Model file for the job. Use its own axes, mm. Coordinates: 2 decimals unless noted, no trailing zeros. Write each loop counter-clockwise with the first axis right and the second up, starting at its lowest first coordinate (ties: lowest second). Pieces come first, ordered by that corner, then holes. Notation, with made-up numbers: (-30, 69.5) - (-5, 69.5) arc R7 cw to (-5, 81.5) - close; hole circle Ø10 at (82.5, -15). An arc over 180 degrees is marked (long way). Put each result on its own line as item: value. Start each with the question number.
1. Pull direction Z, two halves, no side cores. Call faces 1 (the face through (-244.27, -2.5, -39.93)), 2 (the face through (-250.948, -2.504, -31.747)), 3 (the face through (-250, 0, -51)): released by +Z, released by -Z, zero draft, split by the parting line, or undercut.
2. Drop flat-ended pins along their axis: P1, Ø4, axis at x = -254.15, z = -32.75, coming from the +Y side; P2, Ø3, axis at x = -239.5, y = -1, coming from the -Z side. Give the stop position or say it passes through.
3. Saw through at D-D, the plane z = -48. Write the cut outline in (x, y), plus the area to 3 significant figures.
4. Saw through at B-B, the plane z = -33.5. Write the cut outline in (x, y).
5. Drill centre lines: L1, parallel to Z at x = -255.5, y = -1.9; L2, parallel to X at y = -3.25, z = -69.5; L3, parallel to Z at x = -252, y = -3.25. Where is each one in solid material? Low to high. Write a range as from..to.
6. Saw through at A-A, the plane x = -249. Write the cut outline in (y, z).
7. Saw through at C-C, the plane y = -1.4. Write the cut outline in (x, z), plus the area to 3 significant figures.
```python
from build123d import *

# Parameters (mm, degrees)
F0_R     = 16.045413
F0_R_2   = 3.352999
F1_DEPTH = 5.08


with BuildPart() as f1:
    # F0 (on Front) → F1 (new body)
    with BuildSketch(Plane.XZ):
        with BuildLine():
            Line((-269.792154, -66.505959), (-268.242146, -61.329008))
            ThreePointArc((-268.242146, -61.329008), (-269.196215, -63.86387), (-269.792154, -66.505959))
        make_face()
        with BuildLine():
            Line((-255.64608, -19.258766), (-268.242146, -61.329008))
            Line((-268.242146, -61.329008), (-269.792154, -66.505959))
            ThreePointArc((-269.792154, -66.505959), (-246.977926, -88.814828), (-233.206555, -60.030735))
            Line((-233.206555, -60.030735), (-255.64608, -19.258766))
        make_face()
        with Locations((-250.397801, -69.492221)):
            Circle(F0_R, mode=Mode.SUBTRACT)
        with Locations((-254.146576, -32.754317)):
            Circle(F0_R_2, mode=Mode.SUBTRACT)
    extrude(amount=F1_DEPTH)


solid = f1.part
```
Final values:
1. face 1: released by +Z
1. face 2: undercut
1. face 3: zero draft
2. P1: passes through
2. P2: stops at z = -86.72
3. outline: (-264.25, -5.08) - (-239.83, -5.08) - (-239.83, 0) - (-264.25, 0) - close
3. area: 124 mm²
4. outline: (-259.91, -5.08) - (-257.42, -5.08) - (-257.42, 0) - (-259.91, 0) - close; (-250.88, -5.08) - (-247.81, -5.08) - (-247.81, 0) - (-250.88, 0) - close
5. L1: z = -88.44..-84.7, -54.28..-35.82, -29.69..-19.52
5. L2: x = -270.02..-266.44, -234.35..-230.77
5. L3: z = -89.05..-85.46, -53.53..-35.33, -30.18..-25.88
6. outline: (-5.08, -89.07) - (0, -89.07) - (0, -85.48) - (-5.08, -85.48) - close; (-5.08, -53.51) - (0, -53.51) - (0, -31.33) - (-5.08, -31.33) - close
7. outline: (-269.79, -66.51) arc R19.62 ccw (long way) to (-233.21, -60.03) - (-255.65, -19.26) - (-268.24, -61.33) arc R19.62 ccw to start; hole circle Ø32.09 at (-250.4, -69.49); hole circle Ø6.71 at (-254.15, -32.75)
7. area: 824 mm²
